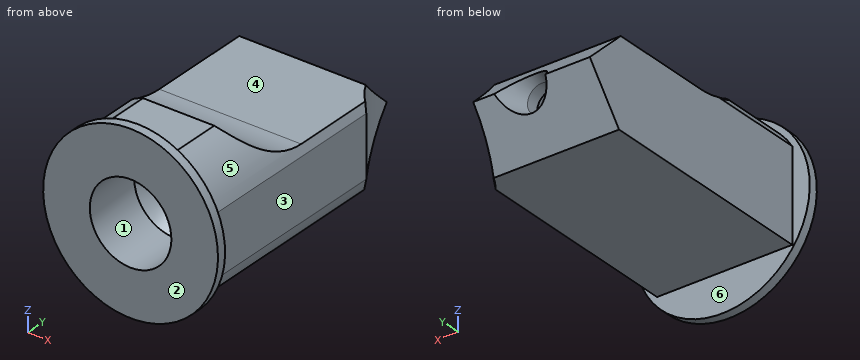
```python
from build123d import *

# Parameters (mm, degrees)
ESBO_O1_R                = 7.5
ESBO_O1_R_2              = 1.25
RESSALTO_EXTRUS_O1_DEPTH = 23.6
CORTE_EXTRUS_O1_START    = -22.8
ESBO_O2_R                = 7.5
CORTE_EXTRUS_O1_DEPTH    = 22.8
CORTE_EXTRUS_O2_DEPTH    = 29.446616671
ESBO_O4_R                = 3.5
ESBO_O4_R_2              = 2.5
ESBO_O4_R_3              = 1.25
CORTE_EXTRUS_O3_DEPTH    = 4
ESBO_O4_3_R              = 2.5
ESBO_O4_3_R_2            = 1.25
CORTE_EXTRUS_O4_DEPTH    = 20
ESBO_O5_R                = 2.2
ESBO_O6_R                = 1.25
ESBO_O7_R                = 7.5
CORTE_EXTRUS_O5_DEPTH    = 28.015736242
CHANFRO1_SIZE            = 2


with BuildPart() as part:
    # Esboço1 → Ressalto-extrusão1 (new body)
    with BuildSketch(Plane(origin=(0, 0, 0), x_dir=(1, 0, 0), z_dir=(0, 1, 0))):
        with Locations(Location((0, 0, 0), (0, 0, 270))):
            Circle(ESBO_O1_R)
        with Locations(Location((0, 0, 0), (0, 0, 270))):
            Circle(ESBO_O1_R_2, mode=Mode.SUBTRACT)
    extrude(amount=RESSALTO_EXTRUS_O1_DEPTH)

    # Esboço2 → Corte-extrusão1 (cut)
    with BuildSketch(Plane(origin=(0, 23.6, 0), x_dir=(1, 0, 0), z_dir=(0, 1, 0)).offset(CORTE_EXTRUS_O1_START)):
        with Locations(Location((0, 0, 0), (0, 0, 270))):
            Circle(ESBO_O2_R)
        with BuildLine():
            ThreePointArc((-6, -3.605551275), (-4.721885351, -5.167571841), (-3.05122926, -6.3))
            Line((-3.05122926, -6.3), (3.05122926, -6.3))
            ThreePointArc((3.05122926, -6.3), (5.121772645, -4.771524386), (6.5, -2.598076211))
            Line((6.5, -2.598076211), (6.5, 2.598076211))
            ThreePointArc((6.5, 2.598076211), (6.102789523, 3.428696552), (5.6, 4.2))
            Line((5.6, 4.2), (-6, 4.2))
            Line((-6, 4.2), (-6, -3.605551275))
        make_face(mode=Mode.SUBTRACT)
    extrude(amount=CORTE_EXTRUS_O1_DEPTH, mode=Mode.SUBTRACT)

    # Esboço3 → Corte-extrusão2 (cut, through all)
    with BuildSketch(Plane(origin=(6.5, 0, 0), x_dir=(0, 0, -1), z_dir=(1, 0, 0))):
        with BuildLine():
            Line((-6.3, 0.8), (-6.3, 5.41))
            ThreePointArc((-6.3, 5.41), (-4.095903015, 7.8849582), (-3.3, 11.102099788))
            Line((-3.3, 11.102099788), (-3.3, 20.102099788))
            Line((-3.3, 20.102099788), (0, 23.6))
            Line((0, 23.6), (4.2, 20.3))
            Line((4.2, 20.3), (4.2, 26.498132866))
            Line((4.2, 26.498132866), (-7.5, 26.498132866))
            Line((-7.5, 26.498132866), (-7.5, 0.8))
            Line((-7.5, 0.8), (-6.3, 0.8))
        make_face()
    extrude(amount=-CORTE_EXTRUS_O2_DEPTH, mode=Mode.SUBTRACT)

    # Esboço4 → Corte-extrusão3 (cut)
    # profile 1 of 2: a face of its own
    with BuildSketch(Plane.XZ):
        with Locations(Location((0, 0, 0), (0, 0, 270))):
            Circle(ESBO_O4_R)
        Circle(ESBO_O4_R_2, mode=Mode.SUBTRACT)
    # profile 2 of 2: a face of its own
    with BuildSketch(Plane.XZ):
        Circle(ESBO_O4_R_2)
        with Locations(Location((0, 0, 0), (0, 0, 270))):
            Circle(ESBO_O4_R_3, mode=Mode.SUBTRACT)
    extrude(amount=-CORTE_EXTRUS_O3_DEPTH, mode=Mode.SUBTRACT)

    # Esboço4<3> → Corte-extrusão4 (cut)
    with BuildSketch(Plane.XZ):
        with Locations(Location((0, 0, 0), (0, 0, 270))):
            Circle(ESBO_O4_3_R)
        with Locations(Location((0, 0, 0), (0, 0, 270))):
            Circle(ESBO_O4_3_R_2, mode=Mode.SUBTRACT)
    extrude(amount=-CORTE_EXTRUS_O4_DEPTH, mode=Mode.SUBTRACT)

    # Esboço5 → Loft de corte1 section 0
    with BuildSketch(Plane(origin=(0, 23.6, 0), x_dir=(1, 0, 0), z_dir=(0, 1, 0))):
        Circle(ESBO_O5_R)
    # Esboço6 → Loft de corte1 section 1
    with BuildSketch(Plane(origin=(0, 21.1, 0), x_dir=(-1, 0, 0), z_dir=(0, -1, 0))):
        Circle(ESBO_O6_R)
    loft(mode=Mode.SUBTRACT)

    # Esboço7 → Corte-extrusão5 (cut, through all)
    with BuildSketch(Plane.XY.offset(3.3)):
        with Locations((11.5, 23.6)):
            Circle(ESBO_O7_R)
    extrude(amount=-CORTE_EXTRUS_O5_DEPTH, mode=Mode.SUBTRACT)

    # Chanfro1
    # the kernel refuses this chamfer: 2 mm, written as the material it takes off along each edge
    with BuildSketch(Plane(origin=(0, 4, 0), x_dir=(0, 0, -1), z_dir=(-1, 0, 0))) as chanfro1_piece_1_section:
        Polygon((2.5 + CHANFRO1_SIZE, 0), (2.5, -CHANFRO1_SIZE), (2.5, 0), align=None)
    chanfro1_piece_1 = revolve(axis=Axis((0, 4, 0), (0, -1, 0)), mode=Mode.PRIVATE)
    chanfro1_piece_1 = chanfro1_piece_1 & Plane(origin=(0, 5.506317811, 0), x_dir=(0, 0, -1), z_dir=(0, -1, 0)) * Cylinder(3.5, 18, mode=Mode.PRIVATE)
    add(chanfro1_piece_1, mode=Mode.SUBTRACT)


solid = part.part
```
Build history of the part. All positions in model axes, mm. Face numbers are marked on the shaded views. A direction names the side the tool comes from. Give positions to 0.01 mm unless a question says otherwise; leave off trailing zeros. Order: outer loops, then holes, each group sorted by start corner. A loop starts at its lowest first (then second) coordinate and runs counter-clockwise, first axis right, second up. Notation, with made-up numbers: M -13.5,-18.5 L 6.5,-18.5 A29 cw 6.5,15.5 Z; hole C -2,-13 d7. An arc over 180 degrees is marked long. Return JSON: item names as keys, results as strings.
Q1. 3-axis set-ups, long thin cutter, end or side, ignore diameter. For the marked faces 4, 5 and 6: which of +Z, -Z, +X, -X, +Y, -Y reach the whole face in a straight line?
Answer list:
{"face 4": "+Z, +X, -X, +Y", "face 5": "+Z, +X, +Y", "face 6": "+Y"}
Q2. Wall check: probe 1 along X at (y, z) = (1.7, 0); probe 2 along Y at (x, z) = (4.5, 5.5); probe 3 along Z at (x, y) = (-0.25, 15.75). Give the ranges that are in metal, low to high. Write a range as from..to.
Answer list:
{"probe 1": "x = -6..-3.5, 3.5..6.5", "probe 2": "y = 0..0.8", "probe 3": "z = -4.2..-2.49, 2.49..3.3"}
Q3. Flat gauge pins, fed straight in: pin 1 (1.6 mm diameter, centred on y = 9.5, z = 0, fed in from +X); pin 2 (3.5 mm diameter, centred on x = -1.5, y = 14.5, fed in from -Z); pin 3 (4.5 mm diameter, centred on x = 1, y = 14.5, fed in from +Z). Where does each tip first touch, or does it go through?
Answer list:
{"pin 1": "stops at x = 6.5", "pin 2": "stops at z = -4.2", "pin 3": "stops at z = 3.3"}
Q4. Band-saw the part on B-B (x = 0). Give the cut face in (y, z), then the cut area to 3 significant figures.
Answer list:
{"outline": "M 0,-7.5 L 0.8,-7.5 L 0.8,-4.2 L 20.3,-4.2 L 22.27,-1.69 L 21.1,-1.25 L 20,-1.25 L 20,-2.5 L 6,-2.5 L 5,-3.5 L 0,-3.5 Z; M 0,3.5 L 5,3.5 L 6,2.5 L 20,2.5 L 20,1.25 L 21.1,1.25 L 21.94,1.57 L 20.1,3.3 L 11.1,3.3 A6.9 cw 5.41,6.3 L 0.8,6.3 L 0.8,7.5 L 0,7.5 Z", "area": "70.1 mm^2"}
Q5. Band-saw the part on D-D (y = 22). Give the cut face in (x, z), then the cut area to 3 significant figures.
Answer list:
{"outline": "M -6,-2.04 L 4.17,-2.04 L 4.17,1.51 L 0.51,1.51 A1.59 cw long -0.51,1.51 L -6,1.51 Z", "area": "28.2 mm^2"}
Q6. Two-plate mould, pull along X, no slides. Class the marked faces 1, 2 and 3: pulls with the +X half, pulls with the -X half, needs draft (parallel to the pull), parting line crosses it, or undercut.
Answer list:
{"face 1": "undercut", "face 2": "needs draft", "face 3": "pulls with the +X half"}
Q7. Band-saw the part on A-A (y = 3.75). Give the cut face in (x, z), then the cut area to 3 significant figures.
Answer list:
{"outline": "M -6,-4.2 L 5.6,-4.2 A7 ccw 6.5,-2.6 L 6.5,2.6 A7 ccw 3.05,6.3 L -3.05,6.3 A7 ccw -6,3.61 Z; hole C 0,0 d7", "area": "84.1 mm^2"}
Q8. Band-saw the part on C-C (z = 6). Give the cut face in (x, y).
Answer list:
{"outline": "M -4.5,0 L 4.5,0 L 4.5,0.8 L 3.61,0.8 L 3.61,5.63 L -3.61,5.63 L -3.61,0.8 L -4.5,0.8 Z"}
